```python
from build123d import *

# Parameters (mm, degrees)
BOSS_EXTRUDE1_DEPTH = 50.8
CUT_EXTRUDE2_START  = -20.32
SKETCH3_R           = 1.27
CUT_EXTRUDE2_DEPTH  = 50.8
CUT_EXTRUDE1_DEPTH  = 50.8
SKETCH4_W           = 10.16
SKETCH4_H           = 15.24
CUT_EXTRUDE3_DEPTH  = 50.8
SKETCH5_R           = 2.54
CUT_EXTRUDE5_DEPTH  = 50.8
CUT_EXTRUDE6_DEPTH  = 32.512
CUT_EXTRUDE7_DEPTH  = 32.512


with BuildPart() as part:
    # Sketch1 → Boss-Extrude1 (new body)
    with BuildSketch(Plane(origin=(0, 0, 0), x_dir=(1, 0, 0), z_dir=(0, 1, 0))):
        with BuildLine():
            Line((-20.32, 27.095319289), (-20.32, 11.855319289))
            ThreePointArc((-20.32, 11.855319289), (-19.204076836, 9.161242453), (-16.51, 8.045319289))
            Line((-16.51, 8.045319289), (-3.81, 8.045319289))
            ThreePointArc((-3.81, 8.045319289), (-1.115923164, 9.161242453), (0, 11.855319289))
            Line((0, 11.855319289), (0, 27.095319289))
            ThreePointArc((0, 27.095319289), (-1.115923164, 29.789396126), (-3.81, 30.905319289))
            Line((-3.81, 30.905319289), (-16.51, 30.905319289))
            ThreePointArc((-16.51, 30.905319289), (-19.204076836, 29.789396126), (-20.32, 27.095319289))
        make_face()
    extrude(amount=BOSS_EXTRUDE1_DEPTH)

    # Sketch3 → Cut-Extrude2 (cut)
    with BuildSketch(Plane(origin=(0, 50.8, 0), x_dir=(1, 0, 0), z_dir=(0, 1, 0)).offset(CUT_EXTRUDE2_START)):
        with Locations(Location((-10.16, 10.585319289, 0), (0, 0, 270))):
            Circle(SKETCH3_R)
        with Locations(Location((-10.16, 28.365319289, 0), (0, 0, 270))):
            Circle(SKETCH3_R)
    extrude(amount=-CUT_EXTRUDE2_DEPTH, mode=Mode.SUBTRACT)

    # Sketch2 → Cut-Extrude1 (cut)
    with BuildSketch(Plane.ZY.offset(20.32)):
        with BuildLine():
            Line((-27.095319289, 7.62), (-30.905319289, 15.24))
            Line((-30.905319289, 15.24), (-30.905319289, -5.08))
            Line((-30.905319289, -5.08), (-8.045319289, -5.08))
            Line((-8.045319289, -5.08), (-8.045319289, 15.24))
            Line((-8.045319289, 15.24), (-11.855319289, 7.62))
            ThreePointArc((-11.855319289, 7.62), (-19.475319289, 0), (-27.095319289, 7.62))
        make_face()
    extrude(amount=-CUT_EXTRUDE1_DEPTH, mode=Mode.SUBTRACT)

    # Sketch4 → Cut-Extrude3 (cut)
    with BuildSketch(Plane.XY.offset(-8.045319289)):
        with Locations((-10.16, 7.62)):
            Rectangle(SKETCH4_W, SKETCH4_H)
    extrude(amount=-CUT_EXTRUDE3_DEPTH, mode=Mode.SUBTRACT)

    # Sketch5 → Cut-Extrude5 (cut)
    with BuildSketch(Plane.ZY.offset(20.32)):
        with Locations((-19.475319289, 7.62)):
            Circle(SKETCH5_R)
    extrude(amount=-CUT_EXTRUDE5_DEPTH, mode=Mode.SUBTRACT)

    # Sketch6 → Cut-Extrude6 (cut)
    with BuildSketch(Plane.ZY.offset(20.32)):
        with BuildLine():
            Line((-11.855319289, 36.846817341), (-21.012334943, 47.93447962))
            ThreePointArc((-21.012334943, 47.93447962), (-23.733254983, 50.047756788), (-27.095319289, 50.8))
            Line((-27.095319289, 50.8), (-31.52544936, 50.8))
            Line((-31.52544936, 50.8), (-31.52544936, 15.08846866))
            Line((-31.52544936, 15.08846866), (-40.392656277, 51.934271372))
            Line((-40.392656277, 51.934271372), (12.273740193, 71.26134954))
            Line((12.273740193, 71.26134954), (-8.045319289, 15.24))
            Line((-8.045319289, 15.24), (-9.357524517, 30.725540243))
            ThreePointArc((-9.357524517, 30.725540243), (-10.139323425, 33.97677891), (-11.855319289, 36.846817341))
        make_face()
    extrude(amount=-CUT_EXTRUDE6_DEPTH, mode=Mode.SUBTRACT)

    # Sketch7 → Cut-Extrude7 (cut)
    with BuildSketch(Plane(origin=(0, 0, -30.905319289), x_dir=(-1, 0, 0), z_dir=(0, 0, -1))):
        with BuildLine():
            Line((0, 29.335182296), (-12.852337187, 67.804770192))
            Line((-12.852337187, 67.804770192), (37.594938904, 66.861563092))
            Line((37.594938904, 66.861563092), (20.32, 29.335182296))
            ThreePointArc((20.32, 29.335182296), (19.06442366, 37.382371637), (16.68228589, 45.170769925))
            ThreePointArc((16.68228589, 45.170769925), (10.662952429, 49.301878805), (4.643618968, 45.170769925))
            ThreePointArc((4.643618968, 45.170769925), (1.994617848, 37.348921605), (0, 29.335182296))
        make_face()
    extrude(amount=-CUT_EXTRUDE7_DEPTH, mode=Mode.SUBTRACT)


solid = part.part
```
Here's how the part is built. I have some questions about the finished solid (model axes, mm). A direction names the side the tool comes from. Give positions to 0.01 mm unless a question says otherwise; leave off trailing zeros. Write each loop counter-clockwise with the first axis right and the second up, starting at its lowest first coordinate (ties: lowest second). Pieces come first, ordered by that corner, then holes. Notation, with made-up numbers: M 68.5,37 L 79.5,37 A28 cw 79.5,59 Z; hole C -32.75,9.25 d2. An arc over 180 degrees is marked long. Put each result on its own line as item: value. Start each with the question number.
Item 1: Will these pins go through, and if not, where does the flat tip stop? pin 1 (11 mm diameter, centred on x = -12, z = -22, fed in from -Y); pin 2 (12 mm diameter, centred on x = -17.5, y = 28.5, fed in from +Z); pin 3 (3 mm diameter, centred on x = -10, z = -11, fed in from -Y); pin 4 (4 mm diameter, centred on x = -10.16, z = -10.59, fed in from +Y).
Item 2: If we section it at C-C, the plane y = 22: Write out the boundary of the cut face in (x, z), then the cut area to 3 significant figures.
Item 3: If we section it at B-B, the plane z = -16.25: Write out the boundary of the cut face in (x, y).
Item 4: If we section it at D-D, the plane z = -24.25: Write out the boundary of the cut face in (x, y), then the cut area to 3 significant figures.
Item 5: On a 3-axis mill with a long thin cutter (end or side, diameter ignored), from which of +Z, -Z, +X, -X, +Y, -Y can I reach the whole of each face in a straight line? I mean faces 1 (the cylindrical face through (-19.174, 26.332, -29.819)), 2 (the flat face through (-10, 15.24, -19)), 3 (the flat face through (-10, 30.48, -11)). Say none if no direction works.
Item 6: I need wall thicknesses on L1, parallel to X at y = 12.5, z = -19.75; L2, parallel to Z at x = -7.75, y = 33.5; L3, parallel to Y at x = -11, z = -25. Which ranges of each line are inside material? Lowest first, please. Write a range as from..to.
Item 7: Thinking about a two-plate mould opening in X: for faces 4 (the cylindrical face through (-10.104, 22.967, -29.634)), 5 (the flat face through (-10.638, 42.313, -16.37)), 6 (the cylindrical face through (-1.086, 25.027, -29.76)), which applies, +X half, -X half, draft (parallel to the pull), parting line (faces both ways), or undercut?
Item 8: If we section it at A-A, the plane y = 16: Write out the boundary of the cut face in (x, z).
Values:
1. pin 1: y = 0
1. pin 2: z = -8.66
1. pin 3: y = 15.24
1. pin 4: y = 37.74
2. outline: M -20.32,-27.1 A3.81 ccw -16.51,-30.91 L -3.81,-30.91 A3.81 ccw 0,-27.1 L 0,-11.86 A3.81 ccw -1.8,-8.62 L -18.52,-8.62 A3.81 ccw -20.32,-11.86 Z; hole C -10.16,-28.37 d2.54; hole C -10.16,-10.59 d2.54
2. area: 433 mm²
3. outline: M -20.32,0.72 L -15.24,0.72 L -15.24,15.24 L -5.08,15.24 L -5.08,0.72 L 0,0.72 L 0,29.34 A100.01 ccw -3.54,42.17 L -17.74,42.17 A57.39 ccw -20.32,29.34 Z
4. outline: M -20.32,1.68 L -15.24,1.68 L -15.24,15.24 L -5.08,15.24 L -5.08,1.68 L 0,1.68 L 0,29.34 A100.01 ccw -4.64,45.17 A6.45 ccw -16.68,45.17 A57.39 ccw -20.32,29.34 Z
4. area: 726 mm²
5. face 1: -Z, -X, +Y, -Y
5. face 2: +Z, -Z, -Y
5. face 3: -Y
6. L1: -20.32..-15.24, -5.08..0
6. L2: -30.91..-9.96
6. L3: 15.24..49.29
7. face 4: undercut
7. face 5: draft
7. face 6: +X half
8. outline: M -20.32,-27.1 A3.81 ccw -16.51,-30.91 L -3.81,-30.91 A3.81 ccw 0,-27.1 L 0,-11.86 A3.81 ccw -3.11,-8.11 L -17.21,-8.11 A3.81 ccw -20.32,-11.86 Z; hole C -10.16,-28.37 d2.54; hole C -10.16,-10.59 d2.54
